The listing builds one solid part. Answer for the finished solid, in the listing's coordinates (mm). Face numbers are marked on the shaded views. Coordinates: 2 decimals unless noted, no trailing zeros. Order: outer loops, then holes, each group sorted by start corner. A loop starts at its lowest first (then second) coordinate and runs counter-clockwise, first axis right, second up. Notation, with made-up numbers: (-29.75, 3) -> (13.25, 3) arc R16 ccw to (13.25, 21) -> close; hole circle Ø4 at (-17.5, 57.25). An arc over 180 degrees is marked (long way). Answer in a Markdown table with one row per item.
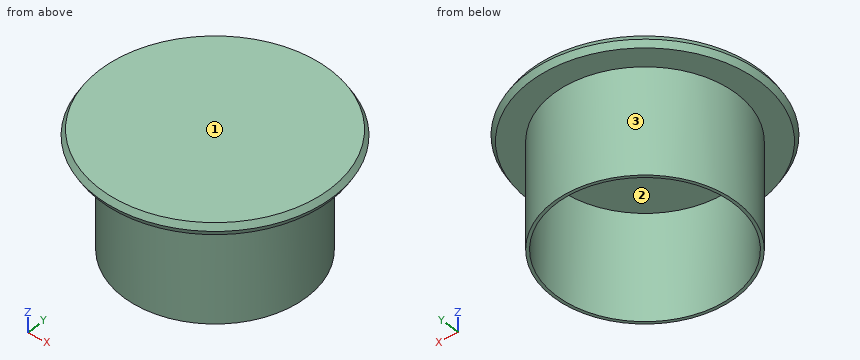
```python
from build123d import *

# Parameters (mm, degrees)
F0_R          = 20
F1_DEPTH      = 1
F1_TAPER      = 30
F1_DEPTH_BACK = 1
F1_TAPER_BACK = 30
F2_R          = 15.5
F2_R_2        = 15
F3_DEPTH      = 18


with BuildPart() as f1:
    # F0 (on Top) → F1 (new body, two sides)
    with BuildSketch(Plane.XY) as f1_sk:
        Circle(F0_R)
    extrude(amount=F1_DEPTH, taper=F1_TAPER)
    extrude(f1_sk.sketch, amount=-F1_DEPTH_BACK, taper=F1_TAPER_BACK)

    # F2 (on face) → F3 (join)
    with BuildSketch(Plane(origin=(0, 0, -1), x_dir=(1, 0, 0), z_dir=(0, 0, -1))):
        Circle(F2_R)
        Circle(F2_R_2, mode=Mode.SUBTRACT)
    extrude(amount=F3_DEPTH)


solid = f1.part
```
(1) A cutting plane is placed at B-B, the plane z = -7.25. Determine the outline of the cut face in (x, y).
Check values:
| item | result |
|---|---|
| outline | circle Ø31 at (0, 0); hole circle Ø30 at (0, 0) |
(2) Find the intervals of material crossed by line 1 along Y through (x, z) = (0, -5); line 2 along Z through (x, y) = (-12, 3), in increasing order. Write a range as from..to.
Check values:
| item | result |
|---|---|
| line 1 | -15.5..-15, 15..15.5 |
| line 2 | -1..1 |
(3) A cutting plane is placed at A-A, the plane x = 0. Determine the outline of the cut face in (y, z), then the cut area to 3 significant figures.
Check values:
| item | result |
|---|---|
| outline | (-20, 0) -> (-19.42, -1) -> (-15.5, -1) -> (-15.5, -19) -> (-15, -19) -> (-15, -1) -> (15, -1) -> (15, -19) -> (15.5, -19) -> (15.5, -1) -> (19.42, -1) -> (20, 0) -> (19.42, 1) -> (-19.42, 1) -> close |
| area | 96.8 mm² |
(4) For a pull along X with two mould halves and no side action, classify the marked faces 1, 2 and 3 as released by +X, released by -X, zero draft, split by the parting line, or undercut.
Check values:
| item | result |
|---|---|
| face 1 | zero draft |
| face 2 | undercut |
| face 3 | split by the parting line |
(5) Flat-ended cylindrical pins translate along their axes: pin 1 (6 mm diameter, centred on y = 6.5, z = -16, fed in from -X); pin 2 (2 mm diameter, centred on x = -7.5, y = -0.5, fed in from -Z); pin 3 (4 mm diameter, centred on y = 8, z = -8, fed in from +X); pin 4 (24 mm diameter, centred on x = -3, y = 3.5, fed in from -Z). Find the tip coordinate at first contact, or state that the pin passes through.
Check values:
| item | result |
|---|---|
| pin 1 | x = -15.1 |
| pin 2 | z = -1 |
| pin 3 | x = 14.29 |
| pin 4 | z = -19 |
